For this review, take the finished solid that the model builds, in its own axes (mm). A direction names the side the tool comes from. Coordinates: 2 decimals unless noted, no trailing zeros. Order: outer loops, then holes, each group sorted by start corner. A loop starts at its lowest first (then second) coordinate and runs counter-clockwise, first axis right, second up. Notation, with made-up numbers: (-37, 69) -> (-22, 69) arc R17 cw to (-22, 76) -> close; hole circle Ø2 at (83.5, -21.5). An arc over 180 degrees is marked (long way). Write item = value, one per line. Start each with the question number.
1) Consider section A-A on x = 10. Give the boundary of the cut face in (y, z).
2) Wall thickness on probe 1 along Y at (x, z) = (9, 3.5); probe 2 along Z at (x, y) = (-13, -1.25); probe 3 along X at (y, z) = (-11.75, 7.5): over which ranges is each line inside the solid? List them lowest first. Write a range as [from, to].
3) Draft analysis for pull direction X (two halves, no side actions). For faces 1 (the face through (39.32, -12.98, 6.26)), 2 (the face through (-8.88, -12.42, 6.44)), 3 (the face through (-19, -18, 38.1)), state which applies: +X half, -X half, draft (parallel to the pull), parting line (faces both ways), or undercut.
4) Insertion check: pin 1 Ø8 at (x, z) = (31.5, 11) entering from -Y; pin 2 Ø7.5 at (x, y) = (16, -10) entering from +Z; pin 3 Ø5 at (y, z) = (-12.5, 17.5) entering from +X. Each pin has a flat end and moves straight along its axis. Give the tip position at first contact, or say it passes through.
5) Consider section D-D on z = 14. Give the boundary of the cut face in (x, y), and give its area (3 significant figures).
6) Consider section C-C on y = -11. Give the boundary of the cut face in (x, z).
7) Consider section B-B on z = 9.5. Give the boundary of the cut face in (x, y), and give its area (3 significant figures).
8) Machinability: for faces 4 (the face through (-36.874, -12.421, 18.783)), 5 (the face through (10, -19.05, 6)), which of the approach directions +Z, -Z, +X, -X, +Y, -Y give a long, thin tool a straight path to every point of the face, cutting with its end or side? Answer none if there is none.
from build123d import *

# Parameters (mm, degrees)
F0_W     = 50.8
F0_H     = 25.4
F1_DEPTH = 12.7
F3_DEPTH = 25.4
F4_R     = 6.512394
F5_DEPTH = 38.1
F7_DEPTH = 12.7


with BuildPart() as f1:
    # F0 (on Top) → F1 (new body)
    with BuildSketch(Plane.XY):
        with Locations((1.222458, -12.7)):
            Rectangle(F0_W, F0_H)
        with BuildLine():
            Line((-24.177542, -25.4), (-24.177542, 0))
            ThreePointArc((-24.177542, 0), (-36.877542, -12.7), (-24.177542, -25.4))
        make_face()
        with BuildLine():
            ThreePointArc((26.622458, -25.4), (39.322458, -12.7), (26.622458, 0))
            Line((26.622458, 0), (26.622458, -25.4))
        make_face()
    extrude(amount=F1_DEPTH)

    # F2 (on face) → F3 (join)
    with BuildSketch(Plane.XY.offset(12.7)):
        with BuildLine():
            ThreePointArc((-22.280858, -25.4), (-14.450198, -21.082493), (-11.336692, -12.7))
            ThreePointArc((-11.336692, -12.7), (-14.450198, -4.317507), (-22.280858, 0))
            Line((-22.280858, 0), (-24.177542, 0))
            ThreePointArc((-24.177542, 0), (-36.877542, -12.7), (-24.177542, -25.4))
            Line((-24.177542, -25.4), (-22.280858, -25.4))
        make_face()
    extrude(amount=F3_DEPTH)

    # F4 (on face) → F5 (cut)
    with BuildSketch(Plane.XY.offset(38.1)):
        with Locations((-24.177542, -12.7)):
            Circle(F4_R)
    extrude(amount=-F5_DEPTH, mode=Mode.SUBTRACT)

    # F6 (on face) → F7 (cut)
    with BuildSketch(Plane.XY.offset(12.7)):
        with BuildLine():
            ThreePointArc((22.866193, -19.05), (29.216193, -12.7), (22.866193, -6.35))
            Line((22.866193, -6.35), (22.866193, -19.05))
        make_face()
        Polygon((22.866193, -6.35), (-2.269224, -6.35), (-2.533807, -19.05), (22.866193, -19.05), align=None)
        with BuildLine():
            Line((-2.533807, -19.05), (-2.269224, -6.35))
            ThreePointArc((-2.269224, -6.35), (-8.885185, -12.564924), (-2.533807, -19.05))
        make_face()
    extrude(amount=-F7_DEPTH, mode=Mode.SUBTRACT)


solid = f1.part
Answer sheet:
q1.outline = (-25.4, 0) -> (-19.05, 0) -> (-19.05, 12.7) -> (-25.4, 12.7) -> close; (-6.35, 0) -> (0, 0) -> (0, 12.7) -> (-6.35, 12.7) -> close
q2.probe_1 = [-25.4, -19.05], [-6.35, 0]
q2.probe_2 = [0, 12.7]
q2.probe_3 = [-36.84, -30.62], [-17.73, -8.82], [29.14, 39.29]
q3.face_1 = +X half
q3.face_2 = undercut
q3.face_3 = draft
q4.pin_1 = -25.37
q4.pin_2 = 12.7
q4.pin_3 = -11.34
q5.outline = (-24.18, -25.4) -> (-22.28, -25.4) arc R12.84 ccw to (-11.34, -12.7) arc R12.84 ccw to (-22.28, 0) -> (-24.18, 0) arc R12.7 ccw to start; hole circle Ø13.02 at (-24.18, -12.7)
q5.area = 379 mm2
q6.outline = (-36.76, 0) -> (-30.46, 0) -> (-30.46, 38.1) -> (-36.76, 38.1) -> close; (-17.89, 0) -> (-8.66, 0) -> (-8.66, 12.7) -> (-11.45, 12.7) -> (-11.45, 38.1) -> (-17.89, 38.1) -> close; (28.98, 0) -> (39.21, 0) -> (39.21, 12.7) -> (28.98, 12.7) -> close
q7.outline = (-24.18, -25.4) -> (26.62, -25.4) arc R12.7 ccw to (26.62, 0) -> (-24.18, 0) arc R12.7 ccw to start; hole circle Ø13.02 at (-24.18, -12.7); hole (-2.53, -19.05) -> (22.87, -19.05) arc R6.35 ccw to (22.87, -6.35) -> (-2.27, -6.35) arc R6.35 ccw (long way) to start
q7.area = 1,210 mm2
q8.face_4 = +Z, -Z, -X
q8.face_5 = +Z, -Z
